Verification items for this drawing (mm, ordinates from the low corner). Round coordinates to 2 decimals unless told otherwise and drop trailing zeros. Order: outer loops, then holes, each group sorted by start corner. A loop starts at its lowest first (then second) coordinate and runs counter-clockwise, first axis right, second up. Notation, with made-up numbers: (-0.75, 61.5) -> (48.25, 61.5) arc R21 ccw to (48.25, 91.5) -> close; hole circle Ø5 at (72, 80.5). An arc over 180 degrees is marked (long way). Return JSON: item names as keys, results as strings. Group by question number.
Item 1: Sectioned sample at B-B on z = 61. Record the cut outline in (x, y) (1 decimal), plus the area to 3 significant figures.
Item 2: Sectioned sample at D-D on y = 3.5. Give the number of separate pieces and of enclosed holes in the cut face, plus the area to 3 significant figures.
Item 3: Sectioned sample at A-A on x = 65.5. Record the cut outline in (y, z).
Item 4: Scan lines: probe 1 along Z at (x, y) = (68, 3.85); probe 2 along X at (y, z) = (3.35, 13) (1 decimal); probe 3 along X at (y, z) = (1.35, 54) (1 decimal). Record each from-to range of solid material in increasing order. Write a range as from..to.
Item 5: Sectioned sample at C-C on x = 36. Record the cut outline in (y, z), plus the area to 3 significant figures.
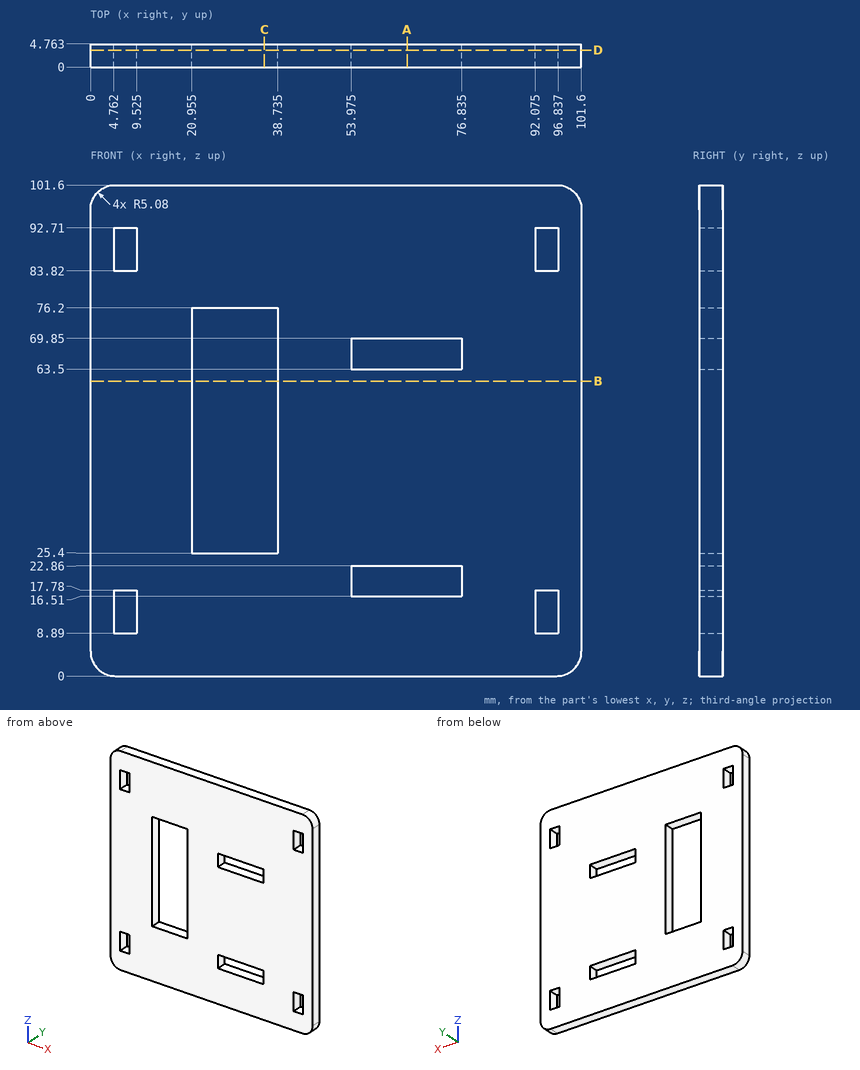
Recorded:
{
 "1": {"outline": "(0, 0) -> (21, 0) -> (21, 4.8) -> (0, 4.8) -> close; (38.7, 0) -> (101.6, 0) -> (101.6, 4.8) -> (38.7, 4.8) -> close", "area": "399 mm²"},
 "2": {"separate pieces": "1", "enclosed holes": "7", "area": "8,940 mm²"},
 "3": {"outline": "(0, 0) -> (4.76, 0) -> (4.76, 16.51) -> (0, 16.51) -> close; (0, 22.86) -> (4.76, 22.86) -> (4.76, 63.5) -> (0, 63.5) -> close; (0, 69.85) -> (4.76, 69.85) -> (4.76, 101.6) -> (0, 101.6) -> close"},
 "4": {"probe 1": "0..16.51, 22.86..63.5, 69.85..101.6", "probe 2": "0..4.8, 9.5..92.1, 96.8..101.6", "probe 3": "0..21, 38.7..101.6"},
 "5": {"outline": "(0, 0) -> (4.76, 0) -> (4.76, 25.4) -> (0, 25.4) -> close; (0, 76.2) -> (4.76, 76.2) -> (4.76, 101.6) -> (0, 101.6) -> close", "area": "242 mm²"}
}
